```python
from build123d import *

# Parameters (mm, degrees)
BOSS_EXTRUDE1_START = 7.62
SKETCH1_R           = 2.4
BOSS_EXTRUDE1_DEPTH = 3.175


with BuildPart() as part:
    # Sketch1 → Boss-Extrude1 (new body)
    with BuildSketch(Plane.XY.offset(BOSS_EXTRUDE1_START)):
        with BuildLine():
            Line((-6.580283468, 85.746774073), (7.851281635, 68.017997221))
            Line((7.851281635, 68.017997221), (22.282846738, 85.746774073))
            ThreePointArc((22.282846738, 85.746774073), (18.702240214, 98.536318224), (7.851281635, 90.877997221))
            ThreePointArc((7.851281635, 90.877997221), (-2.999676943, 98.536318224), (-6.580283468, 85.746774073))
        make_face()
        with Locations((7.851281635, 83.257997221)):
            Circle(SKETCH1_R, mode=Mode.SUBTRACT)
    extrude(amount=BOSS_EXTRUDE1_DEPTH)


solid = part.part
```
Design review of the part built by this model. Coordinates are the model's own, in mm. Round coordinates to 2 decimals unless told otherwise and drop trailing zeros. Order: outer loops, then holes, each group sorted by start corner. A loop starts at its lowest first (then second) coordinate and runs counter-clockwise, first axis right, second up. Notation, with made-up numbers: M 14,86 L 41,86 A24 cw 41,100 Z; hole C 73.5,16.5 d11. An arc over 180 degrees is marked long. Put each result on its own line as item: value.
Q1. Consider section A-A (z = 8.1). State the section outline as (x, y) points, and give its area (3 significant figures).
Reported:
outline: M -6.58,85.75 L 7.85,68.02 L 22.28,85.75 A8.13 ccw long 7.85,90.88 A8.13 ccw long Z; hole C 7.85,83.26 d4.8
area: 606 mm²
Q2. Consider section B-B (y = 88.5). State the section outline as (x, z) points (3 decimals), and give its area (3 significant figures).
Reported:
outline: M -8.049,7.62 L 23.752,7.62 L 23.752,10.795 L -8.049,10.795 Z
area: 101 mm²
Q3. To check wall thickness, follow line 1 (X direction, y = 96, z = 10); line 2 (Y direction, x = 9.5, z = 9.75); line 3 (Y direction, x = 8.5, z = 10.5). State the ranges of each line that lie inside material, in increasing order.
Reported:
line 1: -6.59 to 6.03, 9.67 to 22.29
line 2: 70.04 to 81.51, 85 to 95.79
line 3: 68.81 to 80.95, 85.57 to 94.06
Q4. Consider section C-C (x = 5). State the section outline as (y, z) points (3 decimals).
Reported:
outline: M 71.521,7.62 L 97.06,7.62 L 97.06,10.795 L 71.521,10.795 Z
Q5. Insertion check: pin 1 Ø1.5 at (x, z) = (10, 9) entering from +Y; pin 2 Ø3 at (x, y) = (7.85, 83.26) entering from +Z. Each pin has a flat end and moves straight along its axis. Give the tip position at first contact, or say it passes through.
Reported:
pin 1: y = 97.1
pin 2: through
Q6. Draft analysis for pull direction Y (two halves, no side actions). For faces 1 (the face through (15, 76.8, 9.2)), 2 (the face through (7.539, 85.638, 9.185)), 3 (the face through (8, 87, 7.62)), state which applies: released by +Y, released by -Y, zero draft, split by the parting line, or undercut.
Reported:
face 1: released by -Y
face 2: undercut
face 3: zero draft
